CAD build for the part. Positions are in the model's coordinates, mm. A direction names the side the tool comes from. Round coordinates to 2 decimals unless told otherwise and drop trailing zeros. Order: outer loops, then holes, each group sorted by start corner. A loop starts at its lowest first (then second) coordinate and runs counter-clockwise, first axis right, second up. Notation, with made-up numbers: M -28,-0.5 L -11,-0.5 A18 ccw -11,16.5 Z; hole C 72,0 d9. An arc over 180 degrees is marked long. Answer as a JSON object with one key per item and string values.
```python
from build123d import *

# Parameters (mm, degrees)
EXTRUDE_2_DEPTH     = 1
SKETCH_3_R          = 12
SKETCH_3_R_2        = 11
EXTRUDE_3_DEPTH     = 5
SKETCH_4_R          = 4.5
CUT_EXTRUDE_1_DEPTH = 26.124689053
SKETCH_5_R          = 1.5
CUT_EXTRUDE_2_DEPTH = 26.597851472


with BuildPart() as part:
    # 草图2 → 凸台-拉伸2 (new, symmetric)
    with BuildSketch(Plane.XY):
        with BuildLine():
            Line((-4.5, 12), (4.5, 12))
            ThreePointArc((4.5, 12), (9.857189903, 10.7378078), (14.087412587, 7.216752724))
            ThreePointArc((14.087412587, 7.216752724), (16.191153731, 5.146301215), (18.807692308, 3.780203808))
            ThreePointArc((18.807692308, 3.780203808), (21.5, 0), (18.807692308, -3.780203808))
            ThreePointArc((18.807692308, -3.780203808), (16.191153731, -5.146301215), (14.087412587, -7.216752724))
            ThreePointArc((14.087412587, -7.216752724), (9.857189903, -10.7378078), (4.5, -12))
            Line((4.5, -12), (-4.5, -12))
            ThreePointArc((-4.5, -12), (-9.857189903, -10.7378078), (-14.087412587, -7.216752724))
            ThreePointArc((-14.087412587, -7.216752724), (-16.191153731, -5.146301215), (-18.807692308, -3.780203808))
            ThreePointArc((-18.807692308, -3.780203808), (-21.5, 0), (-18.807692308, 3.780203808))
            ThreePointArc((-18.807692308, 3.780203808), (-16.191153731, 5.146301215), (-14.087412587, 7.216752724))
            ThreePointArc((-14.087412587, 7.216752724), (-9.857189903, 10.7378078), (-4.5, 12))
        make_face()
    extrude(amount=EXTRUDE_2_DEPTH, both=True)

    # 草图3 → 凸台-拉伸3 (add)
    with BuildSketch(Plane.XY.offset(1)):
        with Locations(Location((0, 0, 0), (0, 0, 270))):
            Circle(SKETCH_3_R)
        Circle(SKETCH_3_R_2, mode=Mode.SUBTRACT)
    extrude(amount=EXTRUDE_3_DEPTH)

    # 草图4 → 切除-拉伸1 (cut, through all)
    with BuildSketch(Plane.XY.offset(1)):
        Circle(SKETCH_4_R)
    extrude(amount=-CUT_EXTRUDE_1_DEPTH, mode=Mode.SUBTRACT)

    # 草图5 → 切除-拉伸2 (cut, through all)
    with BuildSketch(Plane(origin=(0, 0, -1), x_dir=(-1, 0, 0), z_dir=(0, 0, -1))):
        with Locations((17.5, 0)):
            Circle(SKETCH_5_R)
        with Locations((-17.5, 0)):
            Circle(SKETCH_5_R)
    extrude(amount=-CUT_EXTRUDE_2_DEPTH, mode=Mode.SUBTRACT)


solid = part.part
```
Item 1: Saw through at B-B on x = -17.5. List the corners of the cut face in (y, z), and give its area (3 significant figures).
Worked answers:
{"outline": "M -4.34,-1 L -1.5,-1 L -1.5,1 L -4.34,1 Z; M 1.5,-1 L 4.34,-1 L 4.34,1 L 1.5,1 Z", "area": "11.4 mm2"}
Item 2: Saw through at C-C on y = -3. List the corners of the cut face in (x, z).
Worked answers:
{"outline": "M -20.15,-1 L -3.35,-1 L -3.35,1 L -10.58,1 L -10.58,6 L -11.62,6 L -11.62,1 L -20.15,1 Z; M 3.35,-1 L 20.15,-1 L 20.15,1 L 11.62,1 L 11.62,6 L 10.58,6 L 10.58,1 L 3.35,1 Z"}
Item 3: Two-plate mould, pull along X, no slides. Class faces 3 (the cylindrical face through (-16, 0, 0)), 4 (the cylindrical face through (9.79, 10.77, 0.01)), 5 (the cylindrical face through (19, 0, 0)), 6 (the flat face through (-13, 0, 1)): released by +X, released by -X, zero draft, split by the parting line, or undercut.
Worked answers:
{"face 3": "undercut", "face 4": "released by +X", "face 5": "undercut", "face 6": "zero draft"}
Item 4: Wall check: line 1 along Y through (x, z) = (0, -0.35); line 2 along Y through (x, z) = (17.5, 0.45); line 3 along Z through (x, y) = (7.5, -4.5). Give the ranges that are in metal, low to high. Write a range as [from, to].
Worked answers:
{"line 1": "y = [-12, -4.5], [4.5, 12]", "line 2": "y = [-4.34, -1.5], [1.5, 4.34]", "line 3": "z = [-1, 1]"}
Item 5: 3-axis set-ups, long thin cutter, end or side, ignore diameter. For faces 1 (the flat face through (0, -5, 1)), 2 (the flat face through (0, -12, 0)): which of +Z, -Z, +X, -X, +Y, -Y reach the whole face in a straight line?
Worked answers:
{"face 1": "+Z", "face 2": "+Z, -Z, +X, -X, -Y"}
Item 6: Saw through at D-D on y = 5.25. List the corners of the cut face in (x, z).
Worked answers:
{"outline": "M -16.05,-1 L 16.05,-1 L 16.05,1 L 10.79,1 L 10.79,6 L 9.67,6 L 9.67,1 L -9.67,1 L -9.67,6 L -10.79,6 L -10.79,1 L -16.05,1 Z"}
Item 7: Saw through at A-A on y = 0. List the corners of the cut face in (x, z), and give its area (3 significant figures).
Worked answers:
{"outline": "M -21.5,-1 L -19,-1 L -19,1 L -21.5,1 Z; M -16,-1 L -4.5,-1 L -4.5,1 L -11,1 L -11,6 L -12,6 L -12,1 L -16,1 Z; M 4.5,-1 L 16,-1 L 16,1 L 12,1 L 12,6 L 11,6 L 11,1 L 4.5,1 Z; M 19,-1 L 21.5,-1 L 21.5,1 L 19,1 Z", "area": "66.0 mm2"}
Item 8: Drop flat-ended pins along their axis: pin 1 Ø1.5 at (y, z) = (8.5, 5) entering from -X; pin 2 Ø2 at (y, z) = (3, 4) entering from +X. Give the stop position or say it passes through.
Worked answers:
{"pin 1": "stops at x = -9.16", "pin 2": "stops at x = 11.83"}
